Source: CAD feature listing. Evaluate the final solid. Frame: model axes, mm. Face numbers are marked on the shaded views. Coordinates: 2 decimals unless noted, no trailing zeros. Loops run counter-clockwise (first coordinate to the right, second up) from the corner with the lowest first, then second, coordinate; pieces in that order, holes last.
from build123d import *

# Parameters (mm, degrees)
SKETCH1_R           = 2.5
BOSS_EXTRUDE1_DEPTH = 6
SKETCH2_R           = 1.25
CUT_EXTRUDE1_DEPTH  = 10


with BuildPart() as part:
    # Sketch1 → Boss-Extrude1 (new body)
    with BuildSketch(Plane.XY):
        with BuildLine():
            Line((0, 5), (-19, 5))
            ThreePointArc((-19, 5), (-24, 0), (-19, -5))
            Line((-19, -5), (0, -5))
            ThreePointArc((0, -5), (5, 0), (0, 5))
        make_face()
        with Locations((-19, 0)):
            Circle(SKETCH1_R, mode=Mode.SUBTRACT)
        Circle(SKETCH1_R, mode=Mode.SUBTRACT)
    extrude(amount=BOSS_EXTRUDE1_DEPTH)

    # Sketch2 → Cut-Extrude1 (cut)
    with BuildSketch(Plane(origin=(0, 5, 0), x_dir=(1, 0, 0), z_dir=(0, 1, 0))):
        with Locations((0, -3)):
            Circle(SKETCH2_R)
    extrude(amount=-CUT_EXTRUDE1_DEPTH, mode=Mode.SUBTRACT)


solid = part.part
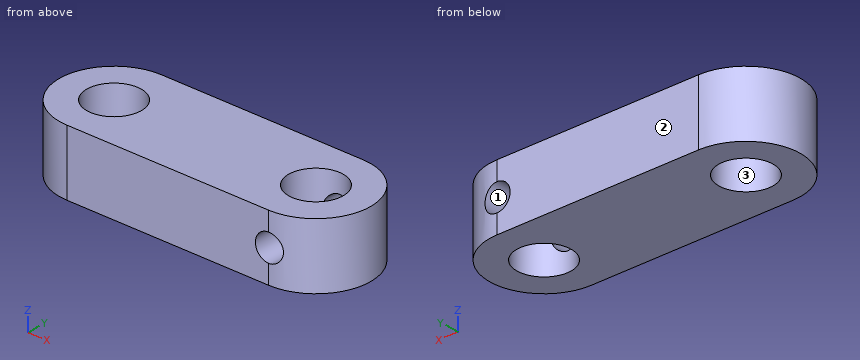
Q1. Contact query for flat-ended pins moving along their axis: pin 1 Ø1.5 at (y, z) = (-3, 2.5) entering from -X; pin 2 Ø4.5 at (x, y) = (-19, 0) entering from +Z. Output: stop coordinate, or through.
Q2. Section A-A, the plane y = 0. Return the cut outline in (x, z), plus the area to 3 significant figures.
Q3. Section C-C, the plane z = 5.25. Return the cut outline in (x, y), plus the area to 3 significant figures.
Q4. Line query: line 1 along Y through (x, z) = (-19, 2.05); line 2 along X through (y, z) = (1, 5.25); line 3 along X through (y, z) = (-1.75, 2.5). Output: solid intervals per line, ascending.
Q5. Section B-B, the plane z = 3. Return the cut outline in (x, y).
Q6. Section D-D, the plane y = -4. Return the cut outline in (x, z).
Q7. Draft query along Y for the marked faces 1, 2 and 3. Return one class per face: +Y half, -Y half, draft (parallel to the pull), parting line (faces both ways), or undercut.
Derived:
1. pin 1: stops at x = -23.47
1. pin 2: passes through
2. outline: (-24, 0) - (-21.5, 0) - (-21.5, 6) - (-24, 6) - close; (-16.5, 0) - (-2.5, 0) - (-2.5, 6) - (-16.5, 6) - close; (2.5, 0) - (5, 0) - (5, 6) - (2.5, 6) - close
2. area: 114 mm2
3. outline: (-19, -5) - (0, -5) arc R5 ccw to (0, 5) - (-19, 5) arc R5 ccw to start; hole circle Ø5 at (-19, 0); hole circle Ø5 at (0, 0)
3. area: 229 mm2
4. line 1: y = -5 to -2.5, 2.5 to 5
4. line 2: x = -23.9 to -21.29, -16.71 to -2.29, 2.29 to 4.9
4. line 3: x = -23.68 to -20.79, -17.21 to -1.79, 1.79 to 4.68
5. outline: (-19, -5) - (-1.25, -5) - (-1.25, -2.17) arc R2.5 cw to (-1.25, 2.17) - (-1.25, 5) - (-19, 5) arc R5 ccw to start; (1.25, -4.84) arc R5 ccw to (1.25, 4.84) - (1.25, 2.17) arc R2.5 cw to (1.25, -2.17) - close; hole circle Ø5 at (-19, 0)
6. outline: (-22, 0) - (3, 0) - (3, 6) - (-22, 6) - close; hole circle Ø2.5 at (0, 3)
7. face 1: draft
7. face 2: +Y half
7. face 3: undercut
